CAD build for the part. Positions are in the model's coordinates, mm. A direction names the side the tool comes from. Give positions to 0.01 mm unless a question says otherwise; leave off trailing zeros. Order: outer loops, then holes, each group sorted by start corner. A loop starts at its lowest first (then second) coordinate and runs counter-clockwise, first axis right, second up.
```python
from build123d import *

# Parameters (mm, degrees)
SKETCH1_R                = 10
BOSS_EXTRUDE1_DEPTH      = 35
SKETCH2_W                = 20
SKETCH2_H                = 30
BOSS_EXTRUDE2_DEPTH      = 35
BOSS_EXTRUDE3_DEPTH      = 80
BOSS_EXTRUDE3_DEPTH_BACK = 80
SKETCH3_W                = 20
SKETCH3_H                = 10
SKETCH4_W                = 20
SKETCH4_H                = 8
BOSS_EXTRUDE4_DEPTH      = 65
SKETCH5_R                = 5
BOSS_EXTRUDE6_DEPTH      = 8
BOSS_EXTRUDE7_START      = -8
SKETCH6_R                = 5
BOSS_EXTRUDE7_DEPTH      = 8
FILLET1_R                = 15
FILLET2_R                = 10
FILLET3_R                = 10
FILLET4_R                = 15
FILLET5_R                = 20
FILLET6_R                = 20
SKETCH7_W                = 12
SKETCH7_H                = 20
CUT_EXTRUDE1_DEPTH       = 30
SKETCH8_R                = 17.5
BOSS_EXTRUDE8_DEPTH      = 30
SKETCH9_R                = 5
CUT_EXTRUDE2_DEPTH       = 20
BOSS_EXTRUDE9_START      = 5
SKETCH10_R               = 15
BOSS_EXTRUDE9_DEPTH      = 5
CUT_EXTRUDE4_START       = -2
SKETCH11_R               = 5
CUT_EXTRUDE4_DEPTH       = 2
CUT_EXTRUDE5_DEPTH       = 211.624072698
FILLET9_R                = 5
BODY_MOVE_COPY1_ANGLE    = 90


with BuildPart() as part:
    # Sketch1 → Boss-Extrude1 (new body)
    with BuildSketch(Plane.XY):
        Circle(SKETCH1_R)
    extrude(amount=BOSS_EXTRUDE1_DEPTH)

    # Sketch2 → Boss-Extrude2 (add)
    with BuildSketch(Plane.XY.offset(35)):
        Rectangle(SKETCH2_W, SKETCH2_H)
    extrude(amount=BOSS_EXTRUDE2_DEPTH)

    # Sketch3 → Boss-Extrude3 (add, two sides: drawn at the far end of the back side and taken through both)
    with BuildSketch(Plane(origin=(0, 0, 0), x_dir=(1, 0, 0), z_dir=(0, 1, 0)).offset(-BOSS_EXTRUDE3_DEPTH_BACK)):
        with Locations((0, -75)):
            Rectangle(SKETCH3_W, SKETCH3_H)
    extrude(amount=BOSS_EXTRUDE3_DEPTH + BOSS_EXTRUDE3_DEPTH_BACK)

    # Sketch4 → Boss-Extrude4 (add)
    with BuildSketch(Plane.XY.offset(80)):
        with Locations((0, 76)):
            Rectangle(SKETCH4_W, SKETCH4_H)
        with Locations((0, -76)):
            Rectangle(SKETCH4_W, SKETCH4_H)
    extrude(amount=BOSS_EXTRUDE4_DEPTH)

    # Sketch5 → Boss-Extrude6 (add)
    with BuildSketch(Plane(origin=(0, 80, 0), x_dir=(1, 0, 0), z_dir=(0, 1, 0))):
        with BuildLine():
            Line((10, -145), (10, -148.819660113))
            ThreePointArc((10, -148.819660113), (0, -175), (-10, -148.819660113))
            Line((-10, -148.819660113), (-10, -145))
            Line((-10, -145), (10, -145))
        make_face()
        with Locations(Location((0, -160, 0), (0, 0, 270))):
            Circle(SKETCH5_R, mode=Mode.SUBTRACT)
    extrude(amount=-BOSS_EXTRUDE6_DEPTH)

    # Sketch6 → Boss-Extrude7 (add)
    with BuildSketch(Plane.XZ.offset(80).offset(BOSS_EXTRUDE7_START)):
        with BuildLine():
            Line((-10, 148.819660113), (-10, 145))
            Line((-10, 145), (10, 145))
            Line((10, 145), (10, 148.819660113))
            ThreePointArc((10, 148.819660113), (0, 175), (-10, 148.819660113))
        make_face()
        with Locations(Location((0, 160, 0), (0, 0, 90))):
            Circle(SKETCH6_R, mode=Mode.SUBTRACT)
    extrude(amount=BOSS_EXTRUDE7_DEPTH)

    # Fillet1
    fillet1_edges = [part.edges().sort_by_distance(p)[0] for p in [
        (0, 80, 70),
    ]]
    fillet(fillet1_edges, radius=FILLET1_R)

    # Fillet2
    fillet2_edges = [part.edges().sort_by_distance(p)[0] for p in [
        (0, 72, 80),
    ]]
    fillet(fillet2_edges, radius=FILLET2_R)

    # Fillet3
    fillet3_edges = [part.edges().sort_by_distance(p)[0] for p in [
        (0, -72, 80),
    ]]
    fillet(fillet3_edges, radius=FILLET3_R)

    # Fillet4
    fillet4_edges = [part.edges().sort_by_distance(p)[0] for p in [
        (0, -80, 70),
    ]]
    fillet(fillet4_edges, radius=FILLET4_R)

    # Fillet5
    fillet5_edges = [part.edges().sort_by_distance(p)[0] for p in [
        (0, 15, 70),
    ]]
    fillet(fillet5_edges, radius=FILLET5_R)

    # Fillet6
    fillet6_edges = [part.edges().sort_by_distance(p)[0] for p in [
        (0, -15, 70),
    ]]
    fillet(fillet6_edges, radius=FILLET6_R)

    # Sketch7 → Cut-Extrude1 (cut)
    with BuildSketch(Plane(origin=(0, 15, 0), x_dir=(1, 0, 0), z_dir=(0, 1, 0))):
        with Locations((0, -60)):
            Rectangle(SKETCH7_W, SKETCH7_H)
    cut_extrude1 = extrude(amount=CUT_EXTRUDE1_DEPTH, mode=Mode.SUBTRACT)

    # Mirror1: Cut-Extrude1 across plane
    add(cut_extrude1.mirror(Plane.ZX), mode=Mode.SUBTRACT)

    # Sketch8 → Boss-Extrude8 (add)
    with BuildSketch(Plane.XZ.offset(80)):
        with Locations(Location((0, 160, 0), (0, 0, 235.150095421))):
            Circle(SKETCH8_R)
    extrude(amount=BOSS_EXTRUDE8_DEPTH)

    # Sketch9 → Cut-Extrude2 (cut)
    with BuildSketch(Plane(origin=(0, -80, 0), x_dir=(1, 0, 0), z_dir=(0, 1, 0))):
        with Locations(Location((0, -160, 0), (0, 0, 270))):
            Circle(SKETCH9_R)
    extrude(amount=-CUT_EXTRUDE2_DEPTH, mode=Mode.SUBTRACT)

    # Sketch10 → Boss-Extrude9 (add)
    with BuildSketch(Plane(origin=(0, 80, 0), x_dir=(1, 0, 0), z_dir=(0, 1, 0)).offset(BOSS_EXTRUDE9_START)):
        with Locations(Location((0, -160, 0), (0, 0, 270))):
            Circle(SKETCH10_R)
    extrude(amount=-BOSS_EXTRUDE9_DEPTH)

    # Sketch11 → Cut-Extrude4 (cut)
    with BuildSketch(Plane.XZ.offset(-80).offset(CUT_EXTRUDE4_START)):
        with Locations(Location((0, 160, 0), (0, 0, 90))):
            Circle(SKETCH11_R)
    extrude(amount=CUT_EXTRUDE4_DEPTH, mode=Mode.SUBTRACT)

    # Sketch12 → Cut-Extrude5 (cut, through all)
    with BuildSketch(Plane(origin=(10, 0, 0), x_dir=(0, 0, -1), z_dir=(1, 0, 0))):
        with BuildLine():
            Line((-73.708886101, 7.5), (-58.708886101, 7.5))
            ThreePointArc((-58.708886101, 7.5), (-51.208886101, 0), (-58.708886101, -7.5))
            Line((-58.708886101, -7.5), (-73.708886101, -7.5))
            Line((-73.708886101, -7.5), (-73.708886101, 7.5))
        make_face()
    extrude(amount=-CUT_EXTRUDE5_DEPTH, mode=Mode.SUBTRACT)

    # Fillet9
    fillet9_edges = [part.edges().sort_by_distance(p)[0] for p in [
        (0, 15, 35),
        (0, -15, 35),
    ]]
    fillet(fillet9_edges, radius=FILLET9_R - 0.0001)  # a hair under: the kernel refuses the full size


with BuildPart() as part_1:
    # Body-Move/Copy1: read off the stored shape, not the designer's step
    # Body-Move/Copy1: moved
    add(part.part.moved(Location((0, 72, -160))).rotate(Axis((0, 0, 0), (0, 1, 0)), BODY_MOVE_COPY1_ANGLE))


solid = part_1.part
```
Item 1: Slice it at A-A (x = 0). Give the cut face in (y, z).
Item 2: Slice it at B-B (z = 12.5). Give the cut face in (x, y).
Item 3: Slice it at C-C (y = 48). Give the cut face in (x, z), and give its area (3 significant figures).
Item 4: Drop flat-ended pins along their axis: pin 1 Ø6 at (y, z) = (56, -13.5) entering from +X; pin 2 Ø12 at (x, z) = (-93, 0) entering from -Y; pin 3 Ø12 at (x, y) = (-82.5, 75.5) entering from +Z; pin 4 Ø6 at (x, z) = (-23, 9.5) entering from +Y. Give the stop position or say it passes through.
Item 5: Two-plate mould, pull along Y, no slides. Class faces 1 (the face through (-125, 81.8, 3)), 2 (the face through (-109, 87, 0)), 3 (the face through (-108.79, 72.16, -0.14)): released by +Y, released by -Y, zero draft, split by the parting line, or undercut.
Item 6: Wall check: L1, parallel to Z at x = 0, y = 148.25; L2, parallel to Y at x = -11, z = 5.5; L3, parallel to X at y = -14, z = 0. Give the ranges that are in metal, low to high.
Item 7: Slice it at D-D (x = -47). Give the cut face in (y, z), and give its area (3 significant figures).
Item 8: Tool access for faces 4 (the face through (14.99, -3.94, -0.51)), 5 (the face through (-86.291, 72, 0)), 6 (the face through (0, 154, 0)): list every direction of +Z, -Z, +X, -X, +Y, -Y with a clear straight run to the whole face (end or side of a thin tool).
A:
1. outline: (-38, -17.5) - (-8, -17.5) - (-8, -15) - (0, -15) - (0, -5) - (-28, -5) - (-28, 5) - (0, 5) - (0, 15) - (-8, 15) - (-8, 17.5) - (-38, 17.5) - close; (144, -15) - (157, -15) - (157, 15) - (144, 15) - (144, 5) - (154, 5) - (154, -5) - (144, -5) - close
2. outline: (-12.25, -38) - (12.25, -38) - (12.25, -8) - (8.29, -8) - (8.29, 0) - (-8.29, 0) - (-8.29, -8) - (-12.25, -8) - close; (-8.29, 144) - (8.29, 144) - (8.29, 157) - (-8.29, 157) - close
3. outline: (-93.3, -10) - (-80, -10) - (-80, 10) - (-93.3, 10) - (-93.3, 6) - (-90, 6) - (-90, -6) - (-93.3, -6) - close
3. area: 226 mm2
4. pin 1: passes through
4. pin 2: stops at y = -2
4. pin 3: stops at z = 10
4. pin 4: stops at y = 152
5. face 1: zero draft
5. face 2: released by +Y
5. face 3: undercut
6. L1: z = -15 to -5, 5 to 15
6. L2: y = -38 to 0, 144 to 157
6. L3: x = -17.5 to -5, 5 to 17.5
7. outline: (-8, -10) - (0, -10) - (0, 10) - (-8, 10) - close; (144, -10) - (152, -10) - (152, 10) - (144, 10) - close
7. area: 320 mm2
8. face 4: +Y
8. face 5: +Z, -Z
8. face 6: none
